from build123d import *

# Parameters (mm, degrees)
BOSS_EXTRUDE1_DEPTH = 5
SKETCH2_R           = 21
CUT_EXTRUDE1_DEPTH  = 8
SKETCH3_R           = 23.2
CUT_EXTRUDE2_DEPTH  = 2.5
BOSS_EXTRUDE2_START = 2.5
BOSS_EXTRUDE2_DEPTH = 2.5


with BuildPart() as part:
    # Sketch1 → Boss-Extrude1 (new body)
    with BuildSketch(Plane(origin=(0, 0, 0), x_dir=(1, 0, 0), z_dir=(0, 1, 0))):
        with BuildLine():
            Line((-30, -40), (30, -40))
            ThreePointArc((30, -40), (37.071067812, -37.071067812), (40, -30))
            Line((40, -30), (40, 30))
            ThreePointArc((40, 30), (37.071067812, 37.071067812), (30, 40))
            Line((30, 40), (-30, 40))
            ThreePointArc((-30, 40), (-37.071067812, 37.071067812), (-40, 30))
            Line((-40, 30), (-40, -30))
            ThreePointArc((-40, -30), (-37.071067812, -37.071067812), (-30, -40))
        make_face()
    extrude(amount=BOSS_EXTRUDE1_DEPTH)

    # Sketch2 → Cut-Extrude1 (cut)
    with BuildSketch(Plane(origin=(0, 5, 0), x_dir=(1, 0, 0), z_dir=(0, 1, 0))):
        with Locations(Location((0, 0, 0), (0, 0, 270))):
            Circle(SKETCH2_R)
    extrude(amount=-CUT_EXTRUDE1_DEPTH, mode=Mode.SUBTRACT)

    # Sketch3 → Cut-Extrude2 (cut)
    with BuildSketch(Plane(origin=(0, 5, 0), x_dir=(1, 0, 0), z_dir=(0, 1, 0))):
        with Locations(Location((0, 0, 0), (0, 0, 270))):
            Circle(SKETCH3_R)
    extrude(amount=-CUT_EXTRUDE2_DEPTH, mode=Mode.SUBTRACT)

    # Sketch4 → Boss-Extrude2 (add)
    with BuildSketch(Plane(origin=(0, 2.5, 0), x_dir=(1, 0, 0), z_dir=(0, 1, 0)).offset(BOSS_EXTRUDE2_START)):
        with BuildLine():
            Line((-22.4, 4), (-22.852570971, 4))
            ThreePointArc((-22.852570971, 4), (-23.112979541, 2.007530008), (-23.2, 0))
            ThreePointArc((-23.2, 0), (-23.112979541, -2.007530008), (-22.852570971, -4))
            Line((-22.852570971, -4), (-22.4, -4))
            Line((-22.4, -4), (-22.4, 4))
        make_face()
        Polygon((23.2, 0), (23.2, 4), (22.4, 4), (22.4, -4), (23.2, -4), align=None)
    extrude(amount=-BOSS_EXTRUDE2_DEPTH)


solid = part.part
Geometry check sheet. Reference: the model listing, model coordinates, mm. A direction names the side the tool comes from. Round coordinates to 2 decimals unless told otherwise and drop trailing zeros. Write each loop counter-clockwise with the first axis right and the second up, starting at its lowest first coordinate (ties: lowest second). Pieces come first, ordered by that corner, then holes. Notation, with made-up numbers: (55, 21.25) -> (112, 21.25) arc R23 cw to (112, 51.25) -> close; hole circle Ø7 at (18.5, 80.25). An arc over 180 degrees is marked (long way). One line per item, written item: value. Start each with the question number.
(1) Cross-section at C-C, the plane y = 3.6. Record the cut outline in (x, z).
(2) Go/stop test with flat-tipped pins: pin 1 Ø1 at (x, z) = (-17, 14.5) entering from +Y; pin 2 Ø2 at (x, y) = (-30.5, 2.5) entering from -Z. Record where each tip stops, or that it passes through.
(3) Draft check along Z on faces 1 (the flat face through (17, 5, -18)), 2 (the flat face through (22.4, 4, 0)), 3 (the cylindrical face through (37.15, 2.46, -36.99)), 4 (the cylindrical face through (-37.15, 2.46, 36.99)). Enter one of: +Z half, -Z half, draft (parallel to the pull), parting line (faces both ways), or undercut.
(4) Cross-section at B-B, the plane z = 0. Record the cut outline in (x, y).
(5) Access from +Z, -Z, +X, -X, +Y, -Y to the whole of each face (thin tool, end or side, straight path). Record for faces 5 (the flat face through (-22.4, 4, 0)), 6 (the flat face through (0, 2, -40)).
(6) Cross-section at A-A, the plane x = 0. Record the cut outline in (y, z).
(7) Scan lines: line 1 (X direction, y = 1.3, z = 0); line 2 (X direction, y = 3.2, z = 0); line 3 (Z direction, x = 15, y = 4.8). Record each from-to range of solid material in increasing order. Write a range as [from, to].
Answer:
1. outline: (-40, -30) arc R10 ccw to (-30, -40) -> (30, -40) arc R10 ccw to (40, -30) -> (40, 30) arc R10 ccw to (30, 40) -> (-30, 40) arc R10 ccw to (-40, 30) -> close; hole (-22.85, -4) arc R23.2 ccw to (22.85, -4) -> (22.4, -4) -> (22.4, 4) -> (22.85, 4) arc R23.2 ccw to (-22.85, 4) -> (-22.4, 4) -> (-22.4, -4) -> close
2. pin 1: y = 2.5
2. pin 2: z = -40
3. face 1: draft
3. face 2: undercut
3. face 3: -Z half
3. face 4: +Z half
4. outline: (-40, 0) -> (-21, 0) -> (-21, 2.5) -> (-22.4, 2.5) -> (-22.4, 5) -> (-40, 5) -> close; (21, 0) -> (40, 0) -> (40, 5) -> (22.4, 5) -> (22.4, 2.5) -> (21, 2.5) -> close
5. face 5: +Y
5. face 6: -Z, +X, -X, +Y, -Y
6. outline: (0, -40) -> (5, -40) -> (5, -23.2) -> (2.5, -23.2) -> (2.5, -21) -> (0, -21) -> close; (0, 21) -> (2.5, 21) -> (2.5, 23.2) -> (5, 23.2) -> (5, 40) -> (0, 40) -> close
7. line 1: [-40, -21], [21, 40]
7. line 2: [-40, -22.4], [22.4, 40]
7. line 3: [-40, -17.7], [17.7, 40]
